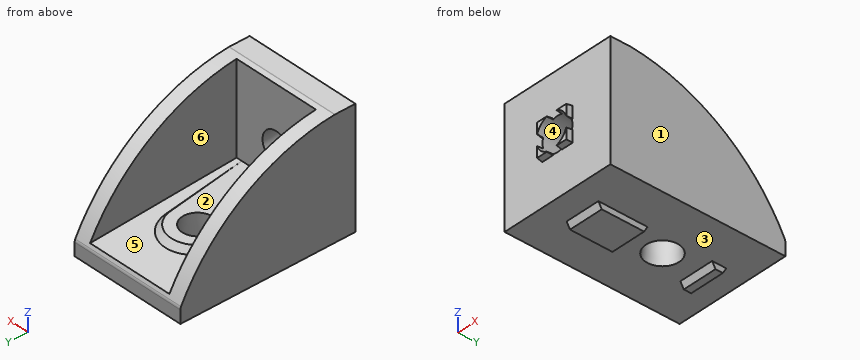
Autodesk Inventor part; units mm, degrees
ref_plane "to_bolt1_XY" through (10, 18, 4.5) normal (0, 0, 1) x (1, 0, 0)
ref_plane "to_bolt1_YZ" through (10, 18, 4.5) normal (1, 0, 0) x (0, 1, 0)
ref_plane "to_bolt1_ZX" through (10, 18, 4.5) normal (0, 1, 0) x (0, 0, 1)
sketch "Sketch_1" plane through (0, 0, 0) normal (1, 0, 0) x (0, 0, -1)
  line L0 (-20, 3.4921) -> (-20, 0)
  line L1 (-20, 0) -> (0, 0)
  line L2 (0, 0) -> (0, 30)
  line L3 (0, 30) -> (-2.2048, 30)
  arc A0 (-2.2048, 30) -> (-2.6607, 29.89) centre (-2.2048, 29) ccw
  arc A1 (-2.6607, 29.89) -> (-19.9977, 3.5593) centre (11.93, 1.41) ccw
  arc A2 (-19.9977, 3.5593) -> (-20, 3.4921) centre (-19, 3.4921) ccw
extrude "Extrusion1" add sketch "Sketch_1" along normal blind 20
sketch "Sketch_2" plane through (10, 0, 0) normal (1, 0, 0) x (0, 0, -1)
  line L0 (-20, 30) -> (-20, 4.5)
  line L1 (-20, 4.5) -> (-4.5, 4.5)
  line L2 (-4.5, 4.5) -> (-3.1636, 30)
  line L3 (-3.1636, 30) -> (-20, 30)
extrude "Extrusion2" cut sketch "Sketch_2" along normal mid plane 15
sketch "Sketch_5" plane through (10, 0, 0) normal (1, 0, 0) x (0, 0, -1)
  line L0 (-0.5, 26.5) -> (-0.5, 23.5)
  line L1 (-0.5, 23.5) -> (1, 24.366)
  line L2 (1, 24.366) -> (1, 25.634)
  line L3 (1, 25.634) -> (-0.5, 26.5)
extrude "Extrusion3" add sketch "Sketch_5" along normal mid plane 6
sketch "Sketch_6" plane through (10, 0, 0) normal (1, 0, 0) x (0, 0, -1)
  line L0 (-0.5, 13) -> (-0.5, 4)
  line L1 (-0.5, 4) -> (1, 4.866)
  line L2 (1, 4.866) -> (1, 12.134)
  line L3 (1, 12.134) -> (-0.5, 13)
extrude "Extrusion4" add sketch "Sketch_6" along normal mid plane 6
sketch "Sketch_3" plane through (0, 0, 4.5) normal (0, 0, 1) x (1, 0, 0)
  line L0 (3.4955, 4.5) -> (16.5045, 4.5)
  line L1 (16.5045, 4.5) -> (14.4534, 18.6457)
  arc A0 (14.4534, 18.6457) -> (5.5466, 18.6457) centre (10, 18) ccw
  line L2 (5.5466, 18.6457) -> (3.4955, 4.5)
extrude "Extrusion5" add sketch "Sketch_3" against normal blind 2 draft 45
sketch "Sketch_7" plane through (0, 0.5, 0) normal (0, 1, 0) x (1, 0, 0)
  line L0 (7.075, -12.925) -> (12.925, -12.925)
  line L1 (12.925, -12.925) -> (12.925, -7.075)
  line L2 (12.925, -7.075) -> (7.075, -7.075)
  line L3 (7.075, -7.075) -> (7.075, -12.925)
extrude "Extrusion6" add sketch "Sketch_7" against normal blind 1.5 draft -6
sketch "Sketch_9" plane through (0, 0, 0) normal (0, 1, 0) x (1, 0, 0)
  line L0 (7.075, -10.835) -> (9.165, -10.835)
  line L1 (9.165, -10.835) -> (9.165, -12.925)
  line L2 (9.165, -12.925) -> (10.835, -12.925)
  line L3 (10.835, -12.925) -> (10.835, -10.835)
  line L4 (10.835, -10.835) -> (12.925, -10.835)
  line L5 (12.925, -10.835) -> (12.925, -9.165)
  line L6 (12.925, -9.165) -> (10.835, -9.165)
  line L7 (10.835, -9.165) -> (10.835, -7.075)
  line L8 (10.835, -7.075) -> (9.165, -7.075)
  line L9 (9.165, -7.075) -> (9.165, -9.165)
  line L10 (9.165, -9.165) -> (7.075, -9.165)
  line L11 (7.075, -9.165) -> (7.075, -10.835)
extrude "Extrusion7" cut sketch "Sketch_9" against normal blind 1 draft 6
sketch "Sketch_4" plane through (10, 0, 0) normal (1, 0, 0) x (0, 0, -1)
  line L0 (0, 18) -> (-4.5, 18)
  line L1 (-4.5, 18) -> (-4.5, 20.6)
  line L2 (-4.5, 20.6) -> (0, 20.8358)
  line L3 (0, 20.8358) -> (0, 18)
  line L4 (0, 18) -> (-4.5, 18)
revolve "Revolution1" cut sketch "Sketch_4" angle 360 about axis through (10, 18, 0) along (0, 0, -1)
sketch "Sketch_8" plane through (10, 0, 0) normal (1, 0, 0) x (0, 0, -1)
  line L0 (-10, -1) -> (-10, 4.5)
  line L1 (-10, 4.5) -> (-7.4, 4.5)
  line L2 (-7.4, 4.5) -> (-7.1118, -1)
  line L3 (-7.1118, -1) -> (-10, -1)
  line L4 (-10, -1) -> (-10, 4.5)
revolve "Revolution2" cut sketch "Sketch_8" angle 360 about axis through (10, -1, 10) along (0, -1, 0)
ref_plane "to_bolt1_XY" through (10, 18, 4.5) normal (0, 0, 1) x (1, 0, 0)
ref_plane "to_bolt1_YZ" through (10, 18, 4.5) normal (1, 0, 0) x (0, 1, 0)
ref_plane "to_bolt1_ZX" through (10, 18, 4.5) normal (0, 1, 0) x (0, 0, 1)
ref_plane "to_bolt2_XY" through (10, 4.5, 10) normal (0, 1, 0) x (1, 0, 0)
ref_plane "to_bolt2_YZ" through (10, 4.5, 10) normal (1, 0, 0) x (0, 0, -1)
ref_plane "to_bolt2_ZX" through (10, 4.5, 10) normal (0, 0, -1) x (0, 1, 0)
ref_plane "to_nut1_XY" through (10, 18, -1) normal (0, 0, -1) x (0, 1, 0)
ref_plane "to_nut1_YZ" through (10, 18, -1) normal (0, 1, 0) x (1, 0, 0)
ref_plane "to_nut1_ZX" through (10, 18, -1) normal (1, 0, 0) x (0, 0, -1)
ref_plane "to_nut2_XY" through (10, -1, 10) normal (0, -1, 0) x (0, 0, -1)
ref_plane "to_nut2_YZ" through (10, -1, 10) normal (0, 0, -1) x (1, 0, 0)
ref_plane "to_nut2_ZX" through (10, -1, 10) normal (1, 0, 0) x (0, -1, 0)
properties part number "HBLFSNF5-SSU_b"
Check sheet for the modelled part. Datum: model origin and axes. Units: mm. Face numbers are marked on the shaded views. A direction names the side the tool comes from. Round coordinates to 2 decimals unless told otherwise and drop trailing zeros. Order: outer loops, then holes, each group sorted by start corner. A loop starts at its lowest first (then second) coordinate and runs counter-clockwise, first axis right, second up.
(1) Go/stop test with flat-tipped pins: P1, Ø4.5, axis at x = 11.5, z = 10, coming from the +Y side; P2, Ø0.5, axis at y = 7.5, z = -0.5, coming from the +X side; P3, Ø1.5, axis at x = 4.5, y = 15, coming from the +Z side. Record where each tip stops, or that it passes through.
(2) Access from +Z, -Z, +X, -X, +Y, -Y to the whole of each face (thin tool, end or side, straight path). Record for the marked faces 1, 2 and 3.
(3) Cross-section at C-C, the plane y = 18. Enter the section's corners in (x, z), and give its area (3 significant figures).
(4) Cross-section at D-D, the plane x = 18.5. Enter the section's corners in (y, z).
(5) Cross-section at A-A, the plane x = 10. Enter the section's corners in (y, z), and give its area (3 significant figures).
(6) Cross-section at B-B, the plane z = 10. Enter the section's corners in (x, y).
(7) Scan lines: probe 1 along X at (y, z) = (7, 12); probe 2 along Z at (x, y) = (8, 14). Record each from-to range of solid material in increasing order.
(8) Draft check along Z on the marked faces 4, 5 and 6. Enter one of: pulls with the +Z half, pulls with the -Z half, needs draft (parallel to the pull), parting line crosses it, or undercut.
Check sheet entries:
1. P1: stops at y = 4.5
1. P2: stops at x = 13
1. P3: stops at z = 4.5
2. face 1: +Z, -Z, +X, +Y, -Y
2. face 2: +Z, +Y
2. face 3: -Z
3. outline: (0, 0) - (7.16, 0) - (7.4, 4.5) - (5.45, 4.5) - (4.74, 3.79) - (2.5, 3.79) - (2.5, 15.43) - (0, 15.43) - close; (12.6, 4.5) - (12.84, 0) - (20, 0) - (20, 15.43) - (17.5, 15.43) - (17.5, 3.79) - (15.26, 3.79) - (14.55, 4.5) - close
3. area: 117 mm2
4. outline: (0, 0) - (30, 0) - (30, 2.2) arc R1 ccw to (29.89, 2.66) arc R32 ccw to (3.56, 20) arc R1.04 ccw to (3.49, 20) - (0, 20) - close
5. outline: (0, 0) - (4.29, 0) - (4.87, -1) - (12.13, -1) - (12.71, 0) - (15.16, 0) - (15.4, 4.5) - (4.5, 4.5) - (4.5, 7.4) - (0, 7.16) - close; (0, 12.84) - (4.5, 12.6) - (4.5, 19.92) arc R32 ccw to (3.56, 20) arc R1.04 ccw to (3.49, 20) - (0, 20) - close; (20.6, 4.5) - (20.84, 0) - (23.79, 0) - (24.37, -1) - (25.63, -1) - (26.21, 0) - (30, 0) - (30, 2.2) arc R1 ccw to (29.89, 2.66) arc R32 ccw to (29.62, 3.18) - (23.5, 3.5) - (22.5, 4.5) - close
5. area: 157 mm2
6. outline: (0, 0) - (7.16, 0) - (7.4, 4.5) - (2.5, 4.5) - (2.5, 24.71) - (0, 24.71) - close; (12.6, 4.5) - (12.84, 0) - (20, 0) - (20, 24.71) - (17.5, 24.71) - (17.5, 4.5) - close
7. probe 1: x = 0 to 2.5, 17.5 to 20
7. probe 2: z = 0 to 4.5
8. face 4: undercut
8. face 5: pulls with the +Z half
8. face 6: needs draft
